```python
from build123d import *

# Parameters (mm, degrees)
BOSS_EXTRUDE1_DEPTH = 127
SHELL1_START        = 2.54
SHELL1_DEPTH        = 121.92
CUT_EXTRUDE5_DEPTH  = 236.549909786
SKETCH20_R          = 3.175
CUT_EXTRUDE7_DEPTH  = 236.549909786
FILLET1_R           = 25.4
SKETCH21_R          = 15.875
SKETCH21_R_2        = 9.525
BOSS_EXTRUDE2_DEPTH = 12.7
SKETCH22_R          = 27.5
SKETCH22_R_2        = 14.2875
BOSS_EXTRUDE4_DEPTH = 1.5875
SKETCH23_R          = 2.5
CUT_EXTRUDE8_DEPTH  = 3.175
SKETCH24_R          = 8.89
CUT_EXTRUDE9_DEPTH  = 12.7
SKETCH25_R          = 15.875
CUT_EXTRUDE10_DEPTH = 63.5
SKETCH26_W          = 7.62
SKETCH26_H          = 35.56
SKETCH26_H_2        = 2.54
BOSS_EXTRUDE5_DEPTH = 31.75
CHAMFER1_SIZE       = 38.1
CHAMFER1_SIZE_2     = 31.969695948
FILLET2_R           = 19.05
SKETCH27_R          = 4.826
CUT_EXTRUDE11_DEPTH = 63.5
SKETCH28_W          = 5
SKETCH28_H          = 60
BOSS_EXTRUDE6_DEPTH = 5
CUT_EXTRUDE13_REACH = 247.036
SKETCH29_R          = 2
SKETCH30_W          = 31.127388046
SKETCH30_H          = 24.370388593
CUT_EXTRUDE14_DEPTH = 12.7
SKETCH31_W          = 38.1
SKETCH31_H          = 2.54
CUT_EXTRUDE15_DEPTH = 30.48


# Read off the part's stored shape, not the designer's step: Shell1
# Some blends are built 0.0001 mm under size
with BuildPart() as part:
    # Sketch3 → Boss-Extrude1 (new body)
    with BuildSketch(Plane(origin=(0, 0, 0), x_dir=(0, 0, -1), z_dir=(1, 0, 0))):
        with BuildLine():
            Line((0, 0), (152.4, 0))
            Line((152.4, 0), (152.4, 97.902234225))
            ThreePointArc((152.4, 97.902234225), (81.095616097, 124.415805368), (35.526445872, 63.5))
            ThreePointArc((35.526445872, 63.5), (-1.951598781, 41.957537243), (-2.199704526, -1.27))
            Line((-2.199704526, -1.27), (0, 0))
        make_face()
    extrude(amount=BOSS_EXTRUDE1_DEPTH)

    # Shell1 outline → Shell1 (cut)
    with BuildSketch(Plane.YZ.offset(SHELL1_START)):
        with BuildLine():
            Line((0, -149.86), (97.146268362, -149.86))
            ThreePointArc((97.146268362, -149.86), (121.481997306, -80.205989224), (60.877364675, -38.122887815))
            ThreePointArc((60.877364675, -38.122887815), (41.799316368, -0.919969929), (0, -9.0799e-05))
            Line((0, -9.0799e-05), (0, -149.86))
        make_face()
    extrude(amount=SHELL1_DEPTH, mode=Mode.SUBTRACT)

    # Sketch19 → Cut-Extrude5 (cut, through all)
    with BuildSketch(Plane(origin=(127, 0, 0), x_dir=(0, 0, -1), z_dir=(1, 0, 0))):
        with BuildLine():
            ThreePointArc((9.525, 12.7), (10.45493597, 10.45493597), (12.7, 9.525))
            Line((12.7, 9.525), (12.7, 12.7))
            Line((12.7, 12.7), (9.525, 12.7))
        make_face()
        with BuildLine():
            Line((12.7, 12.7), (12.7, 9.525))
            ThreePointArc((12.7, 9.525), (14.94506403, 10.45493597), (15.875, 12.7))
            ThreePointArc((15.875, 12.7), (12.7, 15.875), (9.525, 12.7))
            Line((9.525, 12.7), (12.7, 12.7))
        make_face()
    extrude(amount=-CUT_EXTRUDE5_DEPTH, mode=Mode.SUBTRACT)

    # Sketch20 → Cut-Extrude7 (cut, through all)
    with BuildSketch(Plane(origin=(127, 0, 0), x_dir=(0, 0, -1), z_dir=(1, 0, 0))):
        with Locations((63.5, 12.7)):
            Circle(SKETCH20_R)
    extrude(amount=-CUT_EXTRUDE7_DEPTH, mode=Mode.SUBTRACT)

    # Fillet1
    fillet1_edges = [part.edges().sort_by_distance(p)[0] for p in [
        (63.5, 63.5, -35.526445872),
    ]]
    fillet(fillet1_edges, radius=FILLET1_R)

    # Sketch21 → Boss-Extrude2 (add)
    with BuildSketch(Plane(origin=(0, 0, -152.4), x_dir=(-1, 0, 0), z_dir=(0, 0, -1))):
        with Locations(Location((-63.5, 57.384086824, 0), (0, 0, 270))):
            Circle(SKETCH21_R)
        with Locations(Location((-63.5, 57.384086824, 0), (0, 0, 90))):
            Circle(SKETCH21_R_2, mode=Mode.SUBTRACT)
    extrude(amount=BOSS_EXTRUDE2_DEPTH)

    # Sketch22 → Boss-Extrude4 (add, symmetric)
    with BuildSketch(Plane(origin=(0, 0, -165.1), x_dir=(-1, 0, 0), z_dir=(0, 0, -1))):
        with Locations(Location((-63.5, 57.384086824, 0), (0, 0, 90))):
            Circle(SKETCH22_R)
        with Locations(Location((-63.5, 57.384086824, 0), (0, 0, 90))):
            Circle(SKETCH22_R_2, mode=Mode.SUBTRACT)
    extrude(amount=BOSS_EXTRUDE4_DEPTH, both=True)

    # Sketch23 → Cut-Extrude8 (cut)
    with BuildSketch(Plane(origin=(0, 0, -166.6875), x_dir=(-1, 0, 0), z_dir=(0, 0, -1))):
        with Locations(Location((-63.5, 79.884086824, 0), (0, 0, 90))):
            Circle(SKETCH23_R)
        with Locations(Location((-41, 57.384086824, 0), (0, 0, 90))):
            Circle(SKETCH23_R)
        with Locations(Location((-63.5, 34.884086824, 0), (0, 0, 90))):
            Circle(SKETCH23_R)
        with Locations(Location((-86, 57.384086824, 0), (0, 0, 90))):
            Circle(SKETCH23_R)
    extrude(amount=-CUT_EXTRUDE8_DEPTH, mode=Mode.SUBTRACT)

    # Sketch24 → Cut-Extrude9 (cut)
    with BuildSketch(Plane(origin=(0, 0, -152.4), x_dir=(-1, 0, 0), z_dir=(0, 0, -1))):
        with Locations(Location((-63.5, 85.324086824, 0), (0, 0, 90))):
            Circle(SKETCH24_R)
    extrude(amount=-CUT_EXTRUDE9_DEPTH, mode=Mode.SUBTRACT)

    # Sketch25 → Cut-Extrude10 (cut)
    with BuildSketch(Plane.XY):
        with Locations((31.75, 95.25)):
            Circle(SKETCH25_R)
        with Locations((95.25, 95.25)):
            Circle(SKETCH25_R)
    extrude(amount=-CUT_EXTRUDE10_DEPTH, mode=Mode.SUBTRACT)

    # Sketch26 → Boss-Extrude5 (add, symmetric)
    with BuildSketch(Plane.XZ):
        with Locations((40.64, -132.08)):
            Rectangle(SKETCH26_W, SKETCH26_H)
        with Locations((86.36, -132.08)):
            Rectangle(SKETCH26_W, SKETCH26_H)
        with Locations((86.36, -151.13)):
            Rectangle(SKETCH26_W, SKETCH26_H_2)
        with Locations((40.64, -151.13)):
            Rectangle(SKETCH26_W, SKETCH26_H_2)
    extrude(amount=BOSS_EXTRUDE5_DEPTH, both=True)

    # Chamfer1
    # the kernel refuses this chamfer: 38.1, 31.969695948 mm, written as the material it takes off along each edge
    with BuildSketch(Plane(origin=(90.17, 31.75, -114.3), x_dir=(0, 0.024939322090234358, -0.9996889667359941), z_dir=(-1, 0, 0))) as chamfer1_piece_1_section:
        Polygon((CHAMFER1_SIZE * 0.999688966736, CHAMFER1_SIZE * 0.0249393220902), (-CHAMFER1_SIZE_2 * 0.0249393220901, CHAMFER1_SIZE_2 * 0.999688966731), (0, 0), align=None)
    chamfer1_piece_1 = extrude(amount=105.819172537, mode=Mode.PRIVATE)
    chamfer1_piece_1 = split(chamfer1_piece_1, bisect_by=Plane(origin=(86.36, 21.050034317, -149.86), z_dir=(0, 0, 1)), keep=Keep.TOP, mode=Mode.PRIVATE)
    chamfer1_piece_1 = split(chamfer1_piece_1, bisect_by=Plane(origin=(2.54, 21.050034317, -126.894759963), z_dir=(1, 0, 0)), keep=Keep.TOP, mode=Mode.PRIVATE)
    add(chamfer1_piece_1, mode=Mode.SUBTRACT)
    with BuildSketch(Plane(origin=(142.649172537, 31.75, -114.3), x_dir=(0, -0.9993728857116146, 0.03540953691366268), z_dir=(-1, 0, 0))) as chamfer1_piece_2_section:
        Polygon((CHAMFER1_SIZE_2 * 0.999372885707, -CHAMFER1_SIZE_2 * 0.0354095369135), (-CHAMFER1_SIZE * 0.0354095369137, -CHAMFER1_SIZE * 0.999372885712), (0, 0), align=None)
    chamfer1_piece_2 = extrude(amount=204.018345075, mode=Mode.PRIVATE)
    chamfer1_piece_2 = split(chamfer1_piece_2, bisect_by=Plane(origin=(86.36, -0.073231983, -149.86), z_dir=(0, 0, 1)), keep=Keep.TOP, mode=Mode.PRIVATE)
    chamfer1_piece_2 = split(chamfer1_piece_2, bisect_by=Plane(origin=(2.54, -0.073231983, -114.387274478), z_dir=(1, 0, 0)), keep=Keep.TOP, mode=Mode.PRIVATE)
    chamfer1_piece_2 = split(chamfer1_piece_2, bisect_by=Plane(origin=(90.17, -0.073231983, -114.387274478), z_dir=(-1, 0, 0)), keep=Keep.TOP, mode=Mode.PRIVATE)
    add(chamfer1_piece_2, mode=Mode.SUBTRACT)

    # Fillet2
    fillet2_edges = [part.edges().sort_by_distance(p)[0] for p in [
        (86.36, -31.75, -114.3),
        (86.36, -31.75, -152.4),
        (40.64, -31.75, -114.3),
        (40.64, -31.75, -152.4),
    ]]
    fillet(fillet2_edges, radius=FILLET2_R - 0.0001)  # a hair under: the kernel refuses the full size

    # Sketch27 → Cut-Extrude11 (cut)
    with BuildSketch(Plane.ZY.offset(-36.83)):
        with Locations((-133.35, -12.7)):
            Circle(SKETCH27_R)
    extrude(amount=-CUT_EXTRUDE11_DEPTH, mode=Mode.SUBTRACT)

    # Sketch28 → Boss-Extrude6 (add)
    with BuildSketch(Plane.ZY.offset(-124.46)):
        with Locations((-121.96, 30)):
            Rectangle(SKETCH28_W, SKETCH28_H)
        with Locations((-87.844, 30)):
            Rectangle(SKETCH28_W, SKETCH28_H)
    extrude(amount=BOSS_EXTRUDE6_DEPTH)

    # Sketch29 → Cut-Extrude13 (cut, up to next)
    with BuildSketch(Plane(origin=(127, 0, 0), x_dir=(0, 0, -1), z_dir=(1, 0, 0)), mode=Mode.PRIVATE) as cut_extrude13_sk1:
        with Locations((87.844, 52.379999946)):
            Circle(SKETCH29_R)
    cut_extrude13_tool1 = extrude(cut_extrude13_sk1.sketch, amount=-CUT_EXTRUDE13_REACH, mode=Mode.PRIVATE) & part.part
    # Sketch29 → Cut-Extrude13 (cut, up to next)
    with BuildSketch(Plane(origin=(127, 0, 0), x_dir=(0, 0, -1), z_dir=(1, 0, 0)), mode=Mode.PRIVATE) as cut_extrude13_sk2:
        with Locations((87.844, 30.379999946)):
            Circle(SKETCH29_R)
    cut_extrude13_tool2 = extrude(cut_extrude13_sk2.sketch, amount=-CUT_EXTRUDE13_REACH, mode=Mode.PRIVATE) & part.part
    # Sketch29 → Cut-Extrude13 (cut, up to next)
    with BuildSketch(Plane(origin=(127, 0, 0), x_dir=(0, 0, -1), z_dir=(1, 0, 0)), mode=Mode.PRIVATE) as cut_extrude13_sk3:
        with Locations((87.844, 8.281999946)):
            Circle(SKETCH29_R)
    cut_extrude13_tool3 = extrude(cut_extrude13_sk3.sketch, amount=-CUT_EXTRUDE13_REACH, mode=Mode.PRIVATE) & part.part
    # Sketch29 → Cut-Extrude13 (cut, up to next)
    with BuildSketch(Plane(origin=(127, 0, 0), x_dir=(0, 0, -1), z_dir=(1, 0, 0)), mode=Mode.PRIVATE) as cut_extrude13_sk4:
        with Locations((121.92, 52.281999946)):
            Circle(SKETCH29_R)
    cut_extrude13_tool4 = extrude(cut_extrude13_sk4.sketch, amount=-CUT_EXTRUDE13_REACH, mode=Mode.PRIVATE) & part.part
    # Sketch29 → Cut-Extrude13 (cut, up to next)
    with BuildSketch(Plane(origin=(127, 0, 0), x_dir=(0, 0, -1), z_dir=(1, 0, 0)), mode=Mode.PRIVATE) as cut_extrude13_sk5:
        with Locations((121.92, 8.281999946)):
            Circle(SKETCH29_R)
    cut_extrude13_tool5 = extrude(cut_extrude13_sk5.sketch, amount=-CUT_EXTRUDE13_REACH, mode=Mode.PRIVATE) & part.part
    # Sketch29 → Cut-Extrude13 (cut, up to next)
    with BuildSketch(Plane(origin=(127, 0, 0), x_dir=(0, 0, -1), z_dir=(1, 0, 0)), mode=Mode.PRIVATE) as cut_extrude13_sk6:
        with Locations((121.92, 30.281999946)):
            Circle(SKETCH29_R)
    cut_extrude13_tool6 = extrude(cut_extrude13_sk6.sketch, amount=-CUT_EXTRUDE13_REACH, mode=Mode.PRIVATE) & part.part
    add(cut_extrude13_tool1.solids().sort_by_distance((127, 52.38, -87.844))[0], mode=Mode.SUBTRACT)
    add(cut_extrude13_tool2.solids().sort_by_distance((127, 30.38, -87.844))[0], mode=Mode.SUBTRACT)
    add(cut_extrude13_tool3.solids().sort_by_distance((127, 8.282, -87.844))[0], mode=Mode.SUBTRACT)
    add(cut_extrude13_tool4.solids().sort_by_distance((127, 52.282, -121.92))[0], mode=Mode.SUBTRACT)
    add(cut_extrude13_tool5.solids().sort_by_distance((127, 8.282, -121.92))[0], mode=Mode.SUBTRACT)
    add(cut_extrude13_tool6.solids().sort_by_distance((127, 30.282, -121.92))[0], mode=Mode.SUBTRACT)

    # Sketch30 → Cut-Extrude14 (cut)
    with BuildSketch(Plane.ZY.offset(-82.55)):
        with Locations((-115.246305977, 11.965498349)):
            Rectangle(SKETCH30_W, SKETCH30_H)
    extrude(amount=-CUT_EXTRUDE14_DEPTH, mode=Mode.SUBTRACT)

    # Sketch31 → Cut-Extrude15 (cut)
    with BuildSketch(Plane.XZ):
        with Locations((63.5, -151.13)):
            Rectangle(SKETCH31_W, SKETCH31_H)
    extrude(amount=-CUT_EXTRUDE15_DEPTH, mode=Mode.SUBTRACT)


solid = part.part
```
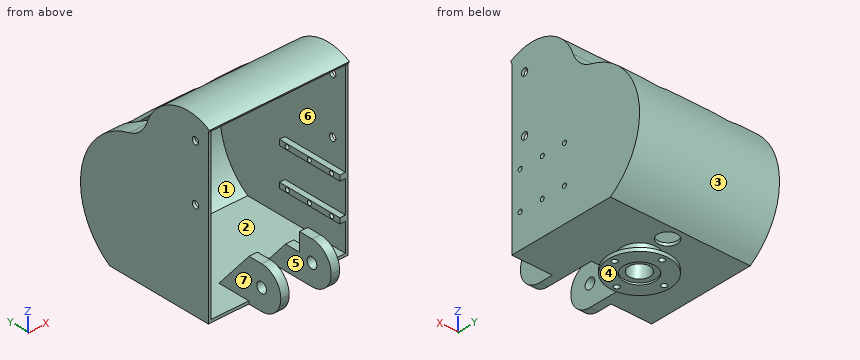
Geometry check sheet. Reference: the model listing, model coordinates, mm. Face numbers are marked on the shaded views. A direction names the side the tool comes from. Coordinates: 2 decimals unless noted, no trailing zeros. Order: outer loops, then holes, each group sorted by start corner. A loop starts at its lowest first (then second) coordinate and runs counter-clockwise, first axis right, second up. Notation, with made-up numbers: (56.5, 29.5) - (64.5, 29.5) arc R20 cw to (64.5, 65.5) - close; hole circle Ø6 at (51, -3). An arc over 180 degrees is marked (long way). Answer in a Markdown table with one row per item. Add a question column.
1. Material ranges on L1, parallel to X at y = 5, z = -50.5; L2, parallel to Z at x = 42, y = -12; L3, parallel to Z at x = 15, y = 70.5, recorded low to high. Write a range as [from, to].
2. Draft check along Z on the marked faces 1, 2, 3 and 4. Enter one of: +Z half, -Z half, draft (parallel to the pull), parting line (faces both ways), or undercut.
3. Access from +Z, -Z, +X, -X, +Y, -Y to the whole of each face (thin tool, end or side, straight path). Record for the marked faces 5, 6 and 7.
4. Gauge pin test, flat ends, axial feed: pin 1 Ø4 at (x, y) = (103, 39.5) entering from +Z; pin 2 Ø3 at (x, y) = (111.5, 82.5) entering from +Z; pin 3 Ø8.5 at (x, y) = (39, -4.5) entering from +Z. Record the tip position at first contact, or that the pin passes through.
5. Section check A-A (z = -72.5). Enter the section's corners in (x, y).
6. Section check B-B (x = 63.5). Give the number of separate pieces and of enclosed holes in the cut face, plus the area to 3 significant figures.
Data:
| question | item | result |
|---|---|---|
| 1 | L1 | x = [0, 2.54], [124.46, 127] |
| 1 | L2 | z = [-152.4, -138.12], [-128.58, -114.3] |
| 1 | L3 | z = [-152.4, -149.86], [-38.47, -33.61] |
| 2 | face 1 | undercut |
| 2 | face 2 | undercut |
| 2 | face 3 | parting line |
| 2 | face 4 | -Z half |
| 3 | face 5 | -Z, -Y |
| 3 | face 6 | none |
| 3 | face 7 | -Y |
| 4 | pin 1 | stops at z = 4.21 |
| 4 | pin 2 | stops at z = -37.99 |
| 4 | pin 3 | stops at z = 2.76 |
| 5 | outline | (0, 0) - (2.54, 0) - (2.54, 118.39) - (124.46, 118.39) - (124.46, 0) - (127, 0) - (127, 121.19) - (0, 121.19) - close |
| 6 | separate pieces | 4 |
| 6 | enclosed holes | 0 |
| 6 | area | 1,020 mm² |
